Design review of the part built by this model. Coordinates are the model's own, in mm. Face numbers are marked on the shaded views. A direction names the side the tool comes from. Give positions to 0.01 mm unless a question says otherwise; leave off trailing zeros. Order: outer loops, then holes, each group sorted by start corner. A loop starts at its lowest first (then second) coordinate and runs counter-clockwise, first axis right, second up. Notation, with made-up numbers: M -4.5,75.5 L 4.5,75.5 A6 cw 4.5,79.5 Z; hole C -22.5,62 d10. An arc over 180 degrees is marked long. Put each result on its own line as item: value. Start each with the question number.
Autodesk Inventor part; units mm, degrees
ref_plane "YZ Plane" through (0, 0, 0) normal (1, 0, 0) x (0, 1, 0)
ref_plane "XZ Plane" through (0, 0, 0) normal (0, 1, 0) x (-1, 0, 0)
ref_plane "XY Plane" through (0, 0, 0) normal (0, 0, 1) x (1, 0, 0)
sketch "Esquisse1" plane through (0, 0, 0) normal (1, 0, 0) x (0, 1, 0)
  circle A0 centre (0, 0) radius 115
  circle A1 centre (0, 0) radius 100
  dimension "d0" = 230
  dimension "d1" = 200
extrude "Extrusion1" add sketch "Esquisse1" along normal blind 270
sketch "Esquisse2" plane through (0, 0, 0) normal (0, 1, 0) x (-1, 0, 0)
  line L0 (-270, 115) -> (-270, -115)
  line L1 (0, -115) -> (-270, -115)
  line L2 (-270, -115) -> (-220, -115)
  line L3 (-220, -115) -> (-220, 115)
  line L4 (-220, 115) -> (-270, 115)
  line L5 (-270, 115) -> (-270, -115)
  point P0 (0, 0)
  point P1 (-270, 0)
  point P2 (-245, -115)
  dimension "d4" = 230
  dimension "d5" = 50
extrude "Extrusion2" cut sketch "Esquisse2" against normal blind 270
sketch "Esquisse3" plane through (0, 0, 0) normal (-1, 0, 0) x (0, 0, 1)
  circle A0 centre (0, 0) radius 115
  circle A1 centre (0, 0) radius 115
  dimension "d8" = 0
extrude "Extrusion3" add sketch "Esquisse3" along normal blind 20
sketch "Esquisse4" plane through (0, 0, 0) normal (1, 0, 0) x (0, 0, -1)
  circle A0 centre (0, 0) radius 115
  dimension "d11" = 230
sketch "Esquisse5" plane through (270, 0, 0) normal (1, 0, 0) x (0, 0, -1)
  circle A0 centre (0, 0) radius 115
  dimension "d12" = 230
extrude "Extrusion4" add sketch "Esquisse5" along normal blind 20
sketch "Esquisse6" plane through (-20, 0, 0) normal (-1, 0, 0) x (0, 0, 1)
  circle A0 centre (0, 0) radius 115
  line L0 (93.037, 67.5953) -> (0, 0)
  line L1 (0, 0) -> (93.037, -67.5953)
  line L2 (0, 0) -> (-35.537, -109.3715)
  arc A1 (-115, 0) -> (115, 0) centre (0, 0) ccw
  line L3 (0, 0) -> (-115, 0)
  line L4 (-100, 0) -> (-115, 0)
  line L5 (0, 0) -> (-35.537, 109.3715)
  circle A2 centre (-57.5, 0) radius 22.5
  circle A3 centre (-17.7685, 54.6857) radius 22.5
  circle A4 centre (46.5185, 33.7977) radius 22.5
  circle A5 centre (46.5185, -33.7977) radius 22.5
  circle A6 centre (-17.7685, -54.6857) radius 22.5
  dimension "d15" = 72
  dimension "d16" = 72
  dimension "d17" = 72
  dimension "d18" = 72
  dimension "d19" = 45
  dimension "d20" = 45
  dimension "d21" = 45
  dimension "d22" = 45
  dimension "d23" = 45
hole "Perçage1" at (-20, 54.6857, -17.7685) at (-20, 33.7977, 46.5185) at (-20, -33.7977, 46.5185) at (-20, -54.6857, -17.7685) at (-20, 0, -57.5) direction (1, 0, 0) diameter 45 depth 40 tip angle 118
properties part number "socle"
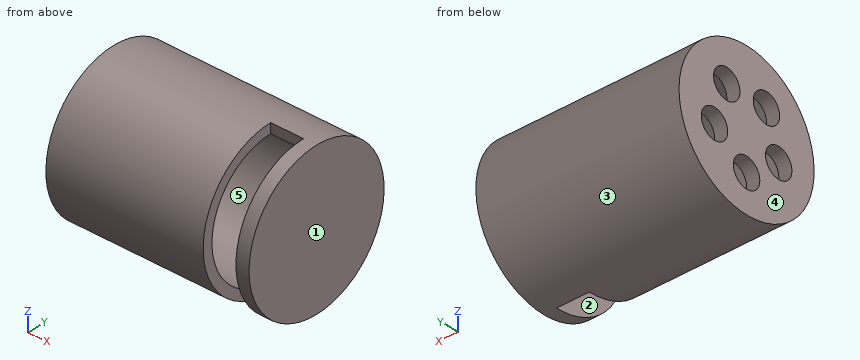
1. Consider section B-B on y = -96. Give the boundary of the cut face in (x, z).
2. To check wall thickness, follow probe 1 along X at (y, z) = (13, -12); probe 2 along Y at (x, z) = (90.5, 0). State the ranges of each line that lie inside material, in increasing order.
3. Machinability: for the marked faces 4 and 5, which of the approach directions +Z, -Z, +X, -X, +Y, -Y give a long, thin tool a straight path to every point of the face, cutting with its end or side? Answer none if there is none.
4. Consider section D-D on x = 140. Give the boundary of the cut face in (y, z), then the cut area to 3 significant figures.
5. The part is to be moulded in two halves that separate along Z. For the marked faces 1, 2 and 3, say which applies: +Z half, -Z half, draft (parallel to the pull), parting line (faces both ways), or undercut.
6. Consider section C-C on y = -65. Give the boundary of the cut face in (x, z).
7. Insertion check: pin 1 (2 mm diameter, centred on x = 189, y = -82, fed in from +Z); pin 2 (1.5 mm diameter, centred on x = 34.5, y = 89, fed in from +Z); pin 3 (16.5 mm diameter, centred on x = 250.5, z = 109.5, fed in from -Y). Each pin has a flat end and moves straight along its axis. Give the tip position at first contact, or say it passes through.
Returned:
1. outline: M -20,-63.32 L 220,-63.32 L 220,-28 L 0,-28 L 0,28 L 220,28 L 220,63.32 L -20,63.32 Z; M 270,-63.32 L 290,-63.32 L 290,63.32 L 270,63.32 Z
2. probe 1: x = -20 to 0, 270 to 290
2. probe 2: y = -115 to -100, 100 to 115
3. face 4: +Z, -Z, -X, +Y, -Y
3. face 5: none
4. outline: C 0,0 d230; hole C 0,0 d200
4. area: 10,100 mm2
5. face 1: draft
5. face 2: undercut
5. face 3: parting line
6. outline: M -20,-94.87 L 220,-94.87 L 220,-75.99 L 0,-75.99 L 0,-37.77 L -20,-37.77 Z; M -20,2.23 L 0,2.23 L 0,75.99 L 220,75.99 L 220,94.87 L -20,94.87 Z; M 270,-94.87 L 290,-94.87 L 290,94.87 L 270,94.87 Z
7. pin 1: stops at z = 81.63
7. pin 2: stops at z = 73.74
7. pin 3: stops at y = 0
